from build123d import *

# Parameters (mm, degrees)
F0_W     = 170
F0_H     = 25
F1_DEPTH = 200
F3_DEPTH = 170.001


with BuildPart() as f1:
    # F0 (on Right) → F1 (new body)
    with BuildSketch(Plane.YZ):
        with Locations((0, 2.5)):
            Rectangle(F0_W, F0_H)
    extrude(amount=-F1_DEPTH)

    # F2 (on face) → F3 (cut, through all)
    with BuildSketch(Plane(origin=(0, 85, 0), x_dir=(-1, 0, 0), z_dir=(0, 1, 0))):
        Polygon((115, 10), (115, 15), (100, 15), (85, 15), (85, 10), (80, 10), (80, 0), (100, 0), (120, 0), (120, 10), align=None)
    extrude(amount=-F3_DEPTH, mode=Mode.SUBTRACT)


solid = f1.part
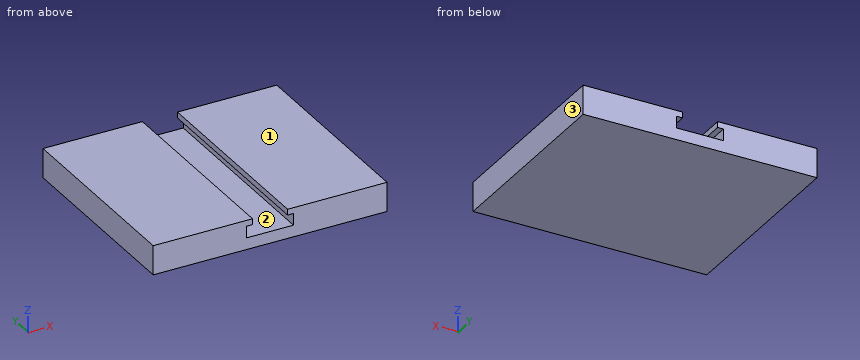
Verification items for the finished model (mm, model axes). Face numbers are marked on the shaded views. Round coordinates to 2 decimals unless told otherwise and drop trailing zeros. Loops run counter-clockwise (first coordinate to the right, second up) from the corner with the lowest first, then second, coordinate; pieces in that order, holes last. Notation, with made-up numbers: (57.25, -15.5) - (114.25, -15.5) arc R18 cw to (114.25, 10.5) - close; hole circle Ø9 at (-6.75, -17.75). An arc over 180 degrees is marked (long way). Answer in a Markdown table with one row per item. Add a question column.
Q1. Release check for a two-part mould opening along Z. For the marked faces 1, 2 and 3 record: pulls with the +Z half, pulls with the -Z half, needs draft (parallel to the pull), parting line crosses it, or undercut.
Q2. Section check C-C on x = -104. Enter the section's corners in (y, z), plus the area to 3 significant figures.
Q3. Section check A-A on z = 2.5. Enter the section's corners in (x, y).
Q4. Material ranges on line 1 (X direction, y = -43, z = 2.25); line 2 (X direction, y = -27, z = 11.75); line 3 (Z direction, x = -118, y = -56.5), recorded low to high.
Q5. Section check B-B on y = 59. Enter the section's corners in (x, z), plus the area to 3 significant figures.
Found:
| question | item | result |
|---|---|---|
| 1 | face 1 | pulls with the +Z half |
| 1 | face 2 | undercut |
| 1 | face 3 | needs draft |
| 2 | outline | (-85, -10) - (85, -10) - (85, 0) - (-85, 0) - close |
| 2 | area | 1,700 mm² |
| 3 | outline | (-200, -85) - (-120, -85) - (-120, 85) - (-200, 85) - close; (-80, -85) - (0, -85) - (0, 85) - (-80, 85) - close |
| 4 | line 1 | x = -200 to -120, -80 to 0 |
| 4 | line 2 | x = -200 to -115, -85 to 0 |
| 4 | line 3 | z = -10 to 0, 10 to 15 |
| 5 | outline | (-200, -10) - (0, -10) - (0, 15) - (-85, 15) - (-85, 10) - (-80, 10) - (-80, 0) - (-120, 0) - (-120, 10) - (-115, 10) - (-115, 15) - (-200, 15) - close |
| 5 | area | 4,450 mm² |
